Geometry check sheet. Reference: the model listing, model coordinates, mm. Coordinates: 2 decimals unless noted, no trailing zeros. Write each loop counter-clockwise with the first axis right and the second up, starting at its lowest first coordinate (ties: lowest second). Pieces come first, ordered by that corner, then holes.
from build123d import *

# Parameters (mm, degrees)
SKETCH_1_W          = 175
SKETCH_1_H          = 166
SKETCH_1_R          = 2
EXTRUDE_1_DEPTH     = 3
SKETCH_2_W          = 12
SKETCH_2_H          = 5
CUT_EXTRUDE_1_DEPTH = 242.226035079
FILLET_1_R          = 2
FILLET_2_R          = 8
SKETCH_4_R          = 1.5
CUT_EXTRUDE_3_DEPTH = 242.226035079


with BuildPart() as part:
    # 草图1 → 凸台-拉伸1 (new body)
    with BuildSketch(Plane(origin=(0, 0, 0), x_dir=(1, 0, 0), z_dir=(0, 1, 0))):
        with Locations((87.5, 83)):
            Rectangle(SKETCH_1_W, SKETCH_1_H)
        with Locations(Location((6, 124.7, 0), (0, 0, 270))):
            Circle(SKETCH_1_R, mode=Mode.SUBTRACT)
        with Locations(Location((6, 69, 0), (0, 0, 270))):
            Circle(SKETCH_1_R, mode=Mode.SUBTRACT)
    extrude(amount=EXTRUDE_1_DEPTH)

    # 草图2 → 切除-拉伸1 (cut, through all)
    with BuildSketch(Plane(origin=(0, 3, 0), x_dir=(1, 0, 0), z_dir=(0, 1, 0))):
        with Locations((169, 131.5)):
            Rectangle(SKETCH_2_W, SKETCH_2_H)
        with Locations((169, 78.5)):
            Rectangle(SKETCH_2_W, SKETCH_2_H)
        with Locations((169, 25.5)):
            Rectangle(SKETCH_2_W, SKETCH_2_H)
    extrude(amount=-CUT_EXTRUDE_1_DEPTH, mode=Mode.SUBTRACT)

    # 圆角1
    fillet_1_edges = [part.edges().sort_by_distance(p)[0] for p in [
        (175, 1.5, -134),
        (175, 1.5, -129),
        (163, 1.5, -129),
        (163, 1.5, -134),
        (175, 1.5, -81),
        (175, 1.5, -76),
        (163, 1.5, -76),
        (163, 1.5, -81),
        (175, 1.5, -28),
        (175, 1.5, -23),
        (163, 1.5, -23),
        (163, 1.5, -28),
    ]]
    fillet(fillet_1_edges, radius=FILLET_1_R)

    # 圆角2
    fillet_2_edges = [part.edges().sort_by_distance(p)[0] for p in [
        (0, 1.5, -166),
        (175, 1.5, -166),
        (175, 1.5, 0),
        (0, 1.5, 0),
    ]]
    fillet(fillet_2_edges, radius=FILLET_2_R)

    # 草图4 → 切除-拉伸3 (cut, through all)
    with BuildSketch(Plane(origin=(0, 3, 0), x_dir=(1, 0, 0), z_dir=(0, 1, 0))):
        with Locations(Location((162.499025796, 10.082661759, 0), (0, 0, 270))):
            Circle(SKETCH_4_R)
        with Locations(Location((169.107894404, 10.082661759, 0), (0, 0, 270))):
            Circle(SKETCH_4_R)
        with Locations(Location((162.499025796, 156.544971591, 0), (0, 0, 270))):
            Circle(SKETCH_4_R)
        with Locations(Location((169.107894404, 156.544971591, 0), (0, 0, 270))):
            Circle(SKETCH_4_R)
    extrude(amount=-CUT_EXTRUDE_3_DEPTH, mode=Mode.SUBTRACT)


solid = part.part
1. Draft check along Z on faces 1 (the cylindrical face through (6.088, 1.479, -126.698)), 2 (the cylindrical face through (2.281, 1.521, -2.406)), 3 (the cylindrical face through (6.601, 1.479, -67.092)), 4 (the cylindrical face through (172.719, 1.521, -163.594)). Enter one of: released by +Z, released by -Z, zero draft, split by the parting line, or undercut.
Computed values:
face 1: undercut
face 2: released by +Z
face 3: undercut
face 4: released by -Z
2. Sectioned sample at B-B, the plane x = 6. Record the boundary of the cut face in (y, z).
Computed values:
outline: (0, -165.75) - (3, -165.75) - (3, -126.7) - (0, -126.7) - close; (0, -122.7) - (3, -122.7) - (3, -71) - (0, -71) - close; (0, -67) - (3, -67) - (3, -0.25) - (0, -0.25) - close
3. Gauge pin test, flat ends, axial feed: pin 1 Ø2.5 at (x, z) = (169.11, -10.08) entering from -Y; pin 2 Ø0.5 at (y, z) = (1, -25.5) entering from +X; pin 3 Ø0.9 at (x, y) = (168.5, 1) entering from +Z; pin 4 Ø0.9 at (x, y) = (169.5, 1) entering from +Z. Record the tip position at first contact, or that the pin passes through.
Computed values:
pin 1: passes through
pin 2: stops at x = 163
pin 3: stops at z = -0.07
pin 4: stops at z = -0.27
4. Thickness scan on line 1 along X through (y, z) = (2.85, -127.5). Record the ranges inside material, lowest first.
Computed values:
line 1: x = 0 to 174.94
5. Sectioned sample at A-A, the plane z = -124.7. Record the boundary of the cut face in (x, y), and give its area (3 significant figures).
Computed values:
outline: (0, 0) - (4, 0) - (4, 3) - (0, 3) - close; (8, 0) - (175, 0) - (175, 3) - (8, 3) - close
area: 513 mm2
